The figure shows three views and two pictorial views of one solid part (mm, origin at its lowest corner). Answer the questions. Round coordinates to 2 decimals unless told otherwise and drop trailing zeros. Order: outer loops, then holes, each group sorted by start corner. A loop starts at its lowest first (then second) coordinate and runs counter-clockwise, first axis right, second up. Notation, with made-up numbers: (6, 32) - (29, 32) arc R21 cw to (29, 64) - close; hole circle Ø6 at (53, 27). An arc over 180 degrees is marked (long way). One line per question, with ' | ' between items. Start each with the question number.
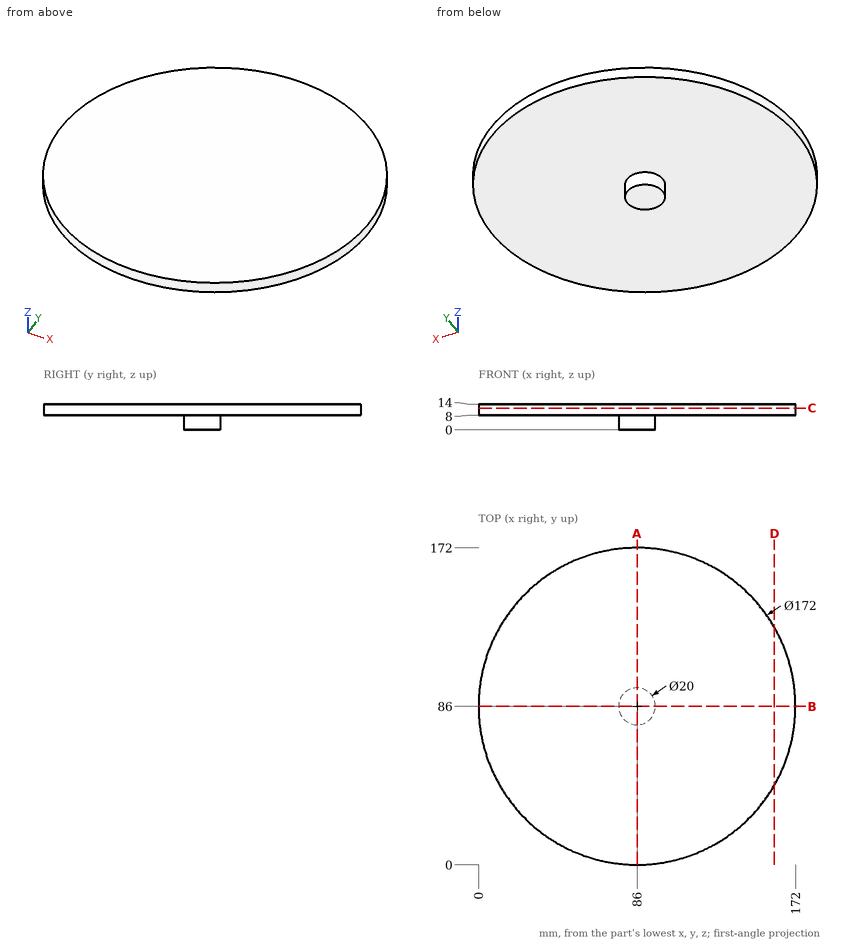
1) Straight lines are drawn through the part: line 1 (Z direction, x = 64.5, y = 118.5); line 2 (X direction, y = 159, z = 9); line 3 (Y direction, x = 25, z = 9.25). For each, find the intervals that lie inside material, in ascending order.
2) Section C-C on z = 11.75 is taken. Give the vertices of the cut face in (x, y).
3) Section D-D on x = 160.5 is taken. Give the vertices of the cut face in (y, z).
4) Section A-A on x = 86 is taken. Give the vertices of the cut face in (y, z), and give its area (3 significant figures).
5) A flat-ended cylindrical pin translates along its axis: pin 1 (10 mm diameter, centred on x = 134, y = 74.5, fed in from -Z). Find the tip coordinate at first contact, or state that the pin passes through.
Recorded:
1) line 1: z = 8 to 14 | line 2: x = 40.54 to 131.46 | line 3: y = 25.38 to 146.62
2) outline: circle Ø172 at (86, 86)
3) outline: (43.04, 8) - (128.96, 8) - (128.96, 14) - (43.04, 14) - close
4) outline: (0, 8) - (76, 8) - (76, 0) - (96, 0) - (96, 8) - (172, 8) - (172, 14) - (0, 14) - close | area: 1,190 mm²
5) pin 1: stops at z = 8
